For this review, take the finished solid that the model builds, in its own axes (mm). Face numbers are marked on the shaded views. A direction names the side the tool comes from. Round coordinates to 2 decimals unless told otherwise and drop trailing zeros. Write each loop counter-clockwise with the first axis right and the second up, starting at its lowest first coordinate (ties: lowest second). Pieces come first, ordered by that corner, then holes.
Solid Edge part; units mm, degrees
sketch "Sketch1" plane through (0, 0, 0) normal (0, -1, 0) x (1, 0, 0)
  line L0 (50, 15) -> (-50, 15)
  line L1 (-50, 15) -> (-50, -15)
  line L2 (-50, -15) -> (50, -15)
  line L3 (50, -15) -> (50, 15)
extrude "Protrusion1" add sketch "Sketch1" against normal blind 20
shell "Thinwall_2" thickness 3 removed faces 1 at (-32.3333, 0, 10.3)
fillet "Round_4" radius 1 8 edges at (0, 17, 12) (0, 17, -12) (-47, 8.5, -12) (-47, 17, 0) (47, 17, 0) (47, 8.5, 12) (47, 8.5, -12) (-47, 8.5, 12)
sketch "Sketch2" plane through (0, 20, 0) normal (0, 1, 0) x (1, 0, 0)
  line L0 (-5, -15.75) -> (5, -15.75)
  line L1 (5, -15.75) -> (5, -14.25)
  line L2 (5, -14.25) -> (-5, -14.25)
  line L3 (-5, -14.25) -> (-5, -15.75)
  line L4 (-5, 14.25) -> (5, 14.25)
  line L5 (5, 14.25) -> (5, 15.75)
  line L6 (5, 15.75) -> (-5, 15.75)
  line L7 (-5, 15.75) -> (-5, 14.25)
extrude "ExtrudedCutout_3" cut sketch "Sketch2" against normal blind 10
sketch "Sketch3" plane through (0, 10, 15) normal (0, 0, 1) x (1, 0, 0)
  line L0 (-5, 9.25) -> (5, 9.25)
  line L1 (5, 9.25) -> (5, 10.75)
  line L2 (5, 10.75) -> (-5, 10.75)
  line L3 (-5, 10.75) -> (-5, 9.25)
extrude "ExtrudedCutout_4" cut sketch "Sketch3" against normal blind 5
sketch "Sketch4" plane through (0, 15, -14.25) normal (0, 0, -1) x (1, 0, 0)
  line L0 (-5, -5.75) -> (5, -5.75)
  line L1 (5, -5.75) -> (5, -4.25)
  line L2 (5, -4.25) -> (-5, -4.25)
  line L3 (-5, -4.25) -> (-5, -5.75)
extrude "ExtrudedCutout_5" cut sketch "Sketch4" against normal blind 5
sketch "Sketch5" plane through (0, 0, 0) normal (0, -1, 0) x (0, 0, 1)
  circle A0 centre (13.5, 0) radius 1
  circle A1 centre (-13.5, 0) radius 1
extrude "ExtrudedCutout_6" cut sketch "Sketch5" against normal blind 8
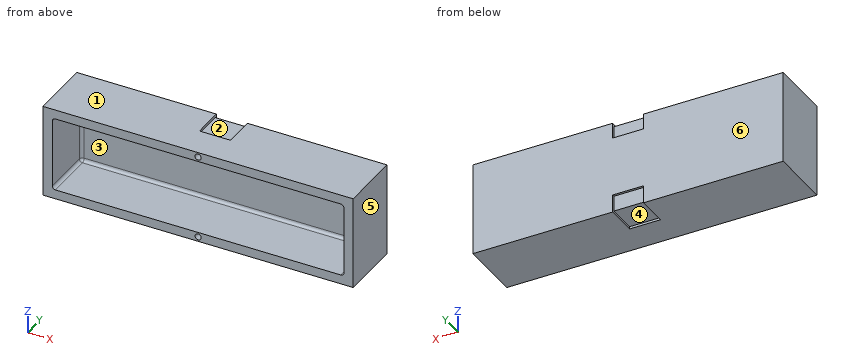
(1) We need section B-B, the plane y = 13. Give the boundary of the cut face in (x, z).
Geometry check:
outline: (-50, -15) - (-5, -15) - (-5, -14.25) - (5, -14.25) - (5, -15) - (50, -15) - (50, 15) - (5, 15) - (5, 14.25) - (-5, 14.25) - (-5, 15) - (-50, 15) - close; hole (-47, -11) arc R1 ccw to (-46, -12) - (46, -12) arc R1 ccw to (47, -11) - (47, 11) arc R1 ccw to (46, 12) - (-46, 12) arc R1 ccw to (-47, 11) - close
(2) We need section A-A, the plane y = 2.5. Give the boundary of the cut face in (x, z), and give its area (3 significant figures).
Geometry check:
outline: (-50, -15) - (50, -15) - (50, 15) - (-50, 15) - close; hole (-47, -11) arc R1 ccw to (-46, -12) - (46, -12) arc R1 ccw to (47, -11) - (47, 11) arc R1 ccw to (46, 12) - (-46, 12) arc R1 ccw to (-47, 11) - close; hole circle Ø2 at (0, -13.5); hole circle Ø2 at (0, 13.5)
area: 739 mm2
(3) Mouldability with a two-part tool opening along X and no side actions: class the marked faces 4, 5 and 6 as pulls with the +X half, pulls with the -X half, needs draft (parallel to the pull), parting line crosses it, or undercut.
Geometry check:
face 4: undercut
face 5: pulls with the +X half
face 6: needs draft
(4) We need section C-C, the plane z = 6.25. Give the boundary of the cut face in (x, y).
Geometry check:
outline: (-50, 0) - (-47, 0) - (-47, 16) arc R1 cw to (-46, 17) - (46, 17) arc R1 cw to (47, 16) - (47, 0) - (50, 0) - (50, 20) - (-50, 20) - close
(5) For pin 1 Ø2.5 at (x, z) = (-2, -12.5) entering from +Y; pin 2 Ø2 at (x, z) = (-27.5, -3) entering from -Y; pin 3 Ø0.8 at (x, y) = (2, 19.5) entering from -Z, all flat-tipped, find the tip position at first contact; note any pin that passes through.
Geometry check:
pin 1: stops at y = 19.25
pin 2: stops at y = 17
pin 3: stops at z = -14.25
(6) We need section D-D, the plane x = 0. Give the boundary of the cut face in (y, z), and give its area (3 significant figures).
Geometry check:
outline: (0, -15) - (10, -15) - (10, -14.25) - (19.25, -14.25) - (19.25, -9.25) - (20, -9.25) - (20, 10) - (19.25, 10) - (19.25, 14.25) - (10, 14.25) - (10, 15) - (0, 15) - (0, 14.5) - (8, 14.5) - (8, 12.5) - (0, 12.5) - (0, 12) - (16, 12) arc R1 cw to (17, 11) - (17, -11) arc R1 cw to (16, -12) - (0, -12) - (0, -12.5) - (8, -12.5) - (8, -14.5) - (0, -14.5) - close
area: 138 mm2
(7) For the marked faces 1, 2 and 3, list the 3-axis set-ups (+Z, -Z, +X, -X, +Y, -Y) from which the entire face can be reached by the end or side of a thin tool; tool diameter is ignored.
Geometry check:
face 1: +Z, +X, -X, +Y, -Y
face 2: +Z, +Y
face 3: -Y
(8) For line 1 along Z through (x, y) = (0, 2.25); line 2 along X through (y, z) = (4, 13.5); line 3 along Z through (x, y) = (3.5, 9.25), list the stretches that pass through material, from the lowest coordinate up.
Geometry check:
line 1: z = -15 to -14.5, -12.5 to -12, 12 to 12.5, 14.5 to 15
line 2: x = -50 to -1, 1 to 50
line 3: z = -15 to -12, 12 to 15
